from build123d import *

# Parameters (mm, degrees)
SKETCH_1_R      = 11.05
SKETCH_1_R_2    = 1.75
EXTRUDE_1_DEPTH = 3
EXTRUDE_2_DEPTH = 3
EXTRUDE_3_DEPTH = 3


with BuildPart() as part:
    # 草图1 → 凸台-拉伸1 (new body)
    with BuildSketch(Plane(origin=(0, 0, 0), x_dir=(1, 0, 0), z_dir=(0, 1, 0))):
        Polygon((-25, 19.5), (-20, 24.5), (20, 24.5), (25, 19.5), (25, -24.5), (-25, -24.5), align=None)
        with Locations(Location((0, 0, 0), (0, 0, 270))):
            Circle(SKETCH_1_R, mode=Mode.SUBTRACT)
        with Locations(Location((15.5, 15.5, 0), (0, 0, 270))):
            Circle(SKETCH_1_R_2, mode=Mode.SUBTRACT)
        with Locations(Location((15.5, -15.5, 0), (0, 0, 270))):
            Circle(SKETCH_1_R_2, mode=Mode.SUBTRACT)
        with Locations(Location((-15.5, -15.5, 0), (0, 0, 270))):
            Circle(SKETCH_1_R_2, mode=Mode.SUBTRACT)
        with Locations(Location((-15.5, 15.5, 0), (0, 0, 270))):
            Circle(SKETCH_1_R_2, mode=Mode.SUBTRACT)
    extrude(amount=EXTRUDE_1_DEPTH)

    # 草图3 → 凸台-拉伸2 (add)
    with BuildSketch(Plane.XY.offset(24.5)):
        Polygon((-25, 3), (25, 3), (25, -43), (20, -48), (-20, -48), (-25, -43), align=None)
        with BuildLine():
            Line((-13.25, -7), (-13.25, -37))
            ThreePointArc((-13.25, -37), (-15, -38.75), (-16.75, -37))
            Line((-16.75, -37), (-16.75, -7))
            ThreePointArc((-16.75, -7), (-15, -5.25), (-13.25, -7))
        make_face(mode=Mode.SUBTRACT)
        with BuildLine():
            Line((13.25, -7), (13.25, -37))
            ThreePointArc((13.25, -37), (15, -38.75), (16.75, -37))
            Line((16.75, -37), (16.75, -7))
            ThreePointArc((16.75, -7), (15, -5.25), (13.25, -7))
        make_face(mode=Mode.SUBTRACT)
    extrude(amount=EXTRUDE_2_DEPTH)

    # 草图4 → 凸台-拉伸3 (add)
    with BuildSketch(Plane(origin=(25, 0, 0), x_dir=(0, 0, -1), z_dir=(1, 0, 0))):
        Polygon((-24.5, 0), (0, 0), (-24.5, -24.5), align=None)
    extrude_3 = extrude(amount=-EXTRUDE_3_DEPTH)

    # 镜向1: 凸台-拉伸3 across plane
    add(extrude_3.mirror(Plane(origin=(0, 0, 0), x_dir=(0, 0, 1), z_dir=(1, 0, 0))))


solid = part.part
Could you check a few things on this model? Use its own coordinates, in mm. A direction names the side the tool comes from. Give positions to 0.01 mm unless a question says otherwise; leave off trailing zeros. Write each loop counter-clockwise with the first axis right and the second up, starting at its lowest first coordinate (ties: lowest second). Pieces come first, ordered by that corner, then holes. Notation, with made-up numbers: (-38, 44.25) -> (-22, 44.25) arc R25 ccw to (-22, 71.25) -> close; hole circle Ø4 at (17, 60.25). An arc over 180 degrees is marked (long way). Answer as CSV lines item,"result". Start each with the question number.
(1) I'm going to push flat-ended pins straight in: pin 1 Ø6 at (x, z) = (-6.5, -17.5) entering from -Y; pin 2 Ø2 at (x, y) = (-17, -13.5) entering from -Z. Where does each tip first touch, or does it pass through?
(2) If we section it at B-B, the plane y = -14.5: Write out the boundary of the cut face in (x, z).
(3) Please list where these lines run through material, in increasing order: line 1 (X direction, y = 1.95, z = -15.5); line 2 (X direction, y = 1.8, z = 0); line 3 (Z direction, x = -15, y = 1).
(4) If we section it at C-C, the plane x = 0: Write out the boundary of the cut face in (y, z).
(5) If we section it at A-A, the plane z = 15.5: Write out the boundary of the cut face in (x, y), and give its area (3 significant figures).
(6) If we mould it in two halves opening along Z, with no side actions, what happens to faces 1 (the face through (-24, -12, 12)), 2 (the face through (25, -8, 14)), 3 (the face through (-10.787, 1.479, -2.395)), 4 (the face through (17.235, 1.479, 15.272))? For each: +Z half, -Z half, draft (parallel to the pull), parting line (faces both ways), or undercut.
(7) Which directions (+Z, -Z, +X, -X, +Y, -Y) give clear straight access to the entire face, cutting with the end or side of a thin tool? Please do faces 5 (the face through (0, -24, 24.5)), 6 (the face through (14.96, -38.75, 25.98)), 7 (the face through (22.5, 1.5, -22)).
(8) If we section it at D-D, the plane z = -15.5: Write out the boundary of the cut face in (x, y).
Answer list:
1,pin 1,"y = 0"
1,pin 2,"z = 24.5"
2,outline,"(-25, 14.5) -> (-22, 14.5) -> (-22, 24.5) -> (-16.75, 24.5) -> (-16.75, 27.5) -> (-25, 27.5) -> close; (-13.25, 24.5) -> (13.25, 24.5) -> (13.25, 27.5) -> (-13.25, 27.5) -> close; (16.75, 24.5) -> (22, 24.5) -> (22, 14.5) -> (25, 14.5) -> (25, 27.5) -> (16.75, 27.5) -> close"
3,line 1,"-25 to -17.25, -13.75 to 13.75, 17.25 to 25"
3,line 2,"-25 to -11.05, 11.05 to 25"
3,line 3,"-24.5 to -17.18, -13.82 to 13.82, 17.18 to 27.5"
4,outline,"(-48, 24.5) -> (0, 24.5) -> (0, 11.05) -> (3, 11.05) -> (3, 27.5) -> (-48, 27.5) -> close; (0, -24.5) -> (3, -24.5) -> (3, -11.05) -> (0, -11.05) -> close"
5,outline,"(-25, -15.5) -> (-22, -15.5) -> (-22, 0) -> (-17.25, 0) -> (-17.25, 3) -> (-25, 3) -> close; (-13.75, 0) -> (13.75, 0) -> (13.75, 3) -> (-13.75, 3) -> close; (17.25, 0) -> (22, 0) -> (22, -15.5) -> (25, -15.5) -> (25, 3) -> (17.25, 3) -> close"
5,area,"222 mm^2"
6,face 1,"-Z half"
6,face 2,"draft"
6,face 3,"undercut"
6,face 4,"undercut"
7,face 5,"-Z, -Y"
7,face 6,"+Z, -Z"
7,face 7,"-Z, +X, +Y, -Y"
8,outline,"(-25, 0) -> (-17.25, 0) -> (-17.25, 3) -> (-25, 3) -> close; (-13.75, 0) -> (13.75, 0) -> (13.75, 3) -> (-13.75, 3) -> close; (17.25, 0) -> (25, 0) -> (25, 3) -> (17.25, 3) -> close"
